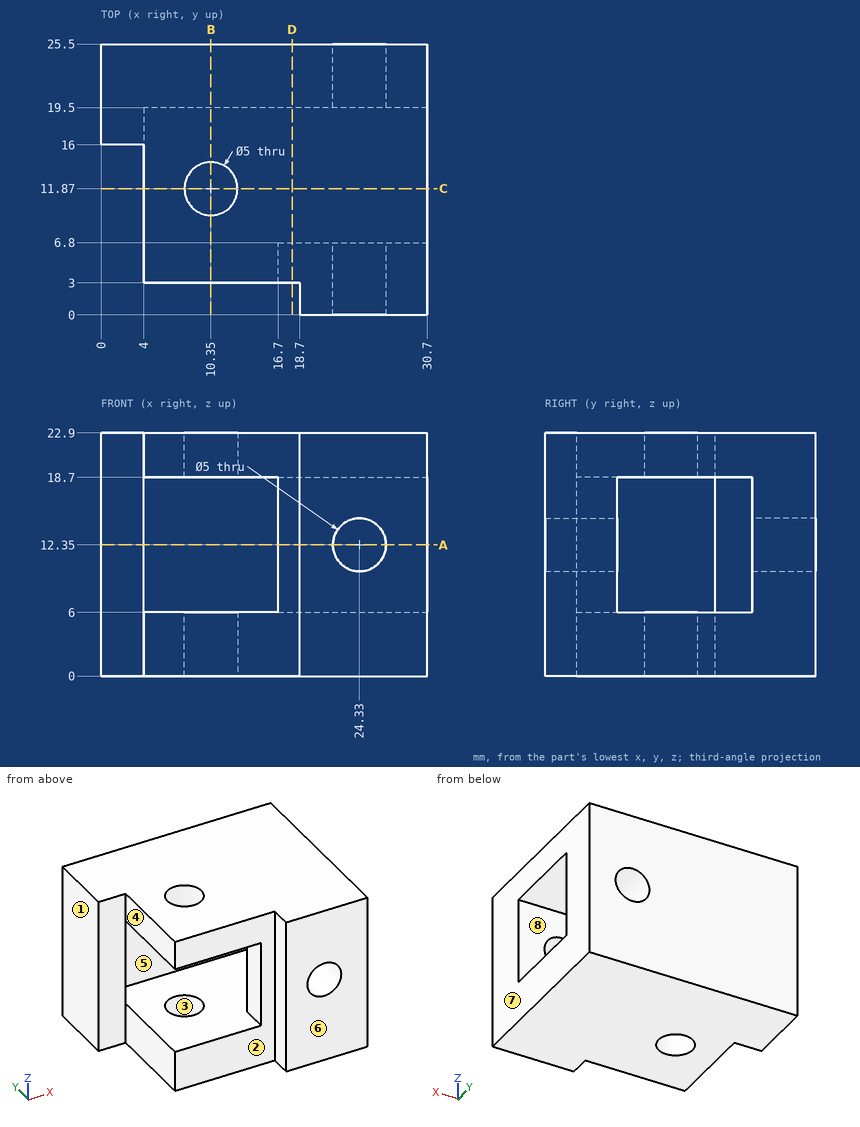
Study the drawing (mm; zero at the part's minimum x, y, z) and answer. A direction names the side the tool comes from. Round coordinates to 2 decimals unless told otherwise and drop trailing zeros. Write each loop counter-clockwise with the first axis right and the second up, starting at its lowest first coordinate (ties: lowest second). Pieces come first, ordered by that corner, then holes. Notation, with made-up numbers: (-26.5, 75.25) -> (-22.5, 75.25) arc R18 ccw to (-22.5, 108.25) -> close; hole circle Ø7 at (-24, 56). An arc over 180 degrees is marked (long way). Write item = value, one per line.
1) Given pin 1 (1.8 mm diameter, centred on y = 8, z = 3.5, fed in from -X); pin 2 (2 mm diameter, centred on x = 2, z = 13, fed in from -Y); pin 3 (1.8 mm diameter, centred on y = 18.5, z = 11.5, fed in from +X); pin 4 (4.5 mm diameter, centred on x = 24.33, z = 12.35, fed in from +Y), each flat-ended and moving along its own axis, determine where each tip first touches the part or whether it passes through.
Check values:
pin_1 = 4
pin_2 = 16
pin_3 = 4
pin_4 = through
2) Which of the six approach directions +Z, -Z, +X, -X, +Y, -Y give full straight-line access (tool end or side, diameter ignored) to the marked faces 4, 5, 6, 7 and 8?
Check values:
face_4 = +Z, -Z, -X, -Y
face_5 = +X
face_6 = +Z, -Z, +X, -X, -Y
face_7 = +Z, -Z, +X, +Y, -Y
face_8 = +X, -X
3) Section C-C on y = 11.87 is taken. Write down the section's boundary in (x, z), plus the area to 3 significant figures.
Check values:
outline = (4, 0) -> (7.85, 0) -> (7.85, 6) -> (4, 6) -> close; (4, 18.7) -> (7.85, 18.7) -> (7.85, 22.9) -> (4, 22.9) -> close; (12.85, 0) -> (30.7, 0) -> (30.7, 6) -> (12.85, 6) -> close; (12.85, 18.7) -> (30.7, 18.7) -> (30.7, 22.9) -> (12.85, 22.9) -> close
area = 221 mm²
4) Section B-B on x = 10.35 is taken. Write down the section's boundary in (y, z).
Check values:
outline = (3, 0) -> (9.37, 0) -> (9.37, 6) -> (3, 6) -> close; (3, 18.7) -> (9.37, 18.7) -> (9.37, 22.9) -> (3, 22.9) -> close; (14.37, 0) -> (25.5, 0) -> (25.5, 22.9) -> (14.37, 22.9) -> (14.37, 18.7) -> (19.5, 18.7) -> (19.5, 6) -> (14.37, 6) -> close
5) Section A-A on z = 12.35 is taken. Write down the section's boundary in (x, y), plus the area to 3 significant figures.
Check values:
outline = (0, 16) -> (4, 16) -> (4, 19.5) -> (21.83, 19.5) -> (21.83, 25.5) -> (0, 25.5) -> close; (16.7, 3) -> (18.7, 3) -> (18.7, 0) -> (21.83, 0) -> (21.83, 6.8) -> (16.7, 6.8) -> close; (26.83, 0) -> (30.7, 0) -> (30.7, 6.8) -> (26.83, 6.8) -> close; (26.83, 19.5) -> (30.7, 19.5) -> (30.7, 25.5) -> (26.83, 25.5) -> close
area = 223 mm²
6) For a pull along X with two mould halves and no side action, classify the marked faces 1, 2 and 3 as released by +X, released by -X, zero draft, split by the parting line, or undercut.
Check values:
face_1 = released by -X
face_2 = zero draft
face_3 = undercut
7) Straight lines are drawn through the part: line 1 along Y through (x, z) = (28, 17.5); line 2 along Z through (x, y) = (8.5, 9.25); line 3 along Y through (x, z) = (10.35, 20.6). For each, find the intervals that lie inside material, in ascending order. Write a range as [from, to].
Check values:
line_1 = [0, 6.8], [19.5, 25.5]
line_2 = [0, 6], [18.7, 22.9]
line_3 = [3, 9.37], [14.37, 25.5]
8) Section D-D on x = 18 is taken. Write down the section's boundary in (y, z).
Check values:
outline = (3, 0) -> (25.5, 0) -> (25.5, 22.9) -> (3, 22.9) -> close; hole (6.8, 6) -> (19.5, 6) -> (19.5, 18.7) -> (6.8, 18.7) -> close
